The model under review builds one solid part; all positions refer to its coordinate system, in mm. Coordinates: 2 decimals unless noted, no trailing zeros. Order: outer loops, then holes, each group sorted by start corner. A loop starts at its lowest first (then second) coordinate and runs counter-clockwise, first axis right, second up. Notation, with made-up numbers: (42, -36.5) - (76, -36.5) arc R19 ccw to (76, -14.5) - close; hole circle Ø2 at (86, 60.5). An arc over 180 degrees is marked (long way). Answer in a Markdown table with one row per item.
```python
from build123d import *

# Parameters (mm, degrees)
F0_R        = 2.286
F1_DEPTH    = 8
F2_R        = 4
F3_R        = 4
F4_T1_DEPTH = 27.7658164516
F5_T1_DEPTH = 27.7658164516


# Not quite as in the source:
# - a fillet or chamfer that OpenCascade refuses, or shapes differently, is made with other operations: its cross-section is extruded or revolved along the edge and cut away or added


with BuildPart() as f1:
    # F0 (on Top) → F1 (new body)
    with BuildSketch(Plane.XY):
        Polygon((19.2099873261, 3.0477390712), (-18.8900126739, 3.0477390712), (-18.8900126739, -3.3271788533), (-17.4405010572, -3.3022609288), (19.2099873261, -3.3022609288), align=None)
        with Locations((-15.8400126739, -0.1272609288)):
            Circle(F0_R, mode=Mode.SUBTRACT)
        with Locations((-7.8400126739, -0.1272609288)):
            Circle(F0_R, mode=Mode.SUBTRACT)
        with Locations((0.1599873261, -0.1272609288)):
            Circle(F0_R, mode=Mode.SUBTRACT)
        with Locations((8.1599873261, -0.1272609288)):
            Circle(F0_R, mode=Mode.SUBTRACT)
        with Locations((16.1599873261, -0.1272609288)):
            Circle(F0_R, mode=Mode.SUBTRACT)
    extrude(amount=F1_DEPTH)

    # F2
    f2_edges = [f1.edges().sort_by_distance(p)[0] for p in [
        (-18.890013, -3.327179, 4),
    ]]
    fillet(f2_edges, radius=F2_R)

    # F3
    f3_edges = [f1.edges().sort_by_distance(p)[0] for p in [
        (19.209987, -3.302261, 4),
    ]]
    fillet(f3_edges, radius=F3_R)

    # F4: fillet of radius 4.5 on 1 edges, made by hand

    # F4_s2 → F4_t1 (cut)
    with BuildSketch(Plane.XY.offset(-9.8829082258)):
        with BuildLine():
            ThreePointArc((19.2099873261, 0.6977390712), (17.5562804933, 2.4158781586), (15.2568240358, 3.0477390712))
            Line((15.2568240358, 3.0477390712), (19.2099873261, 3.0477390712))
            Line((19.2099873261, 3.0477390712), (19.2099873261, 0.6977390712))
        make_face()
    extrude(amount=F4_T1_DEPTH, mode=Mode.SUBTRACT)

    # F5: fillet of radius 4.5 on 1 edges, made by hand

    # F5_s2 → F5_t1 (cut)
    with BuildSketch(Plane.XY.offset(-9.8829082258)):
        with BuildLine():
            ThreePointArc((-18.8900126739, 0.6977390712), (-17.2363058411, 2.4158781586), (-14.9368493836, 3.0477390712))
            Line((-14.9368493836, 3.0477390712), (-18.8900126739, 3.0477390712))
            Line((-18.8900126739, 3.0477390712), (-18.8900126739, 0.6977390712))
        make_face()
    extrude(amount=F5_T1_DEPTH, mode=Mode.SUBTRACT)


solid = f1.part
```
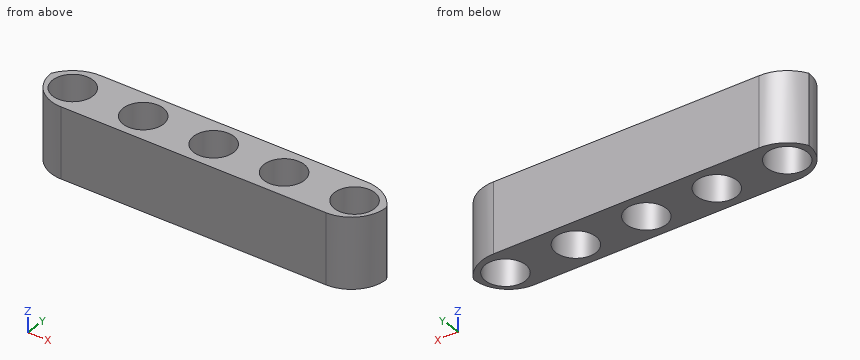
Item 1: We need section B-B, the plane x = -14. Write out the cut boundary in (y, z).
Check values:
| item | result |
|---|---|
| outline | (-3.3, 0) - (-1.48, 0) - (-1.48, 8) - (-3.3, 8) - close; (1.23, 0) - (3.05, 0) - (3.05, 8) - (1.23, 8) - close |
Item 2: We need section C-C, the plane z = 5.5. State how many separate pieces and enclosed holes the cut face has, then the cut area to 3 significant figures.
Check values:
| item | result |
|---|---|
| separate pieces | 1 |
| enclosed holes | 5 |
| area | 148 mm^2 |
Item 3: To check wall thickness, follow line 1 (X direction, y = -1.5, z = 4.75); line 2 (X direction, y = -1.75, z = 5.25); line 3 (Y direction, x = -8, z = 4.5). State the ranges of each line that lie inside material, in increasing order. Write a range as from..to.
Check values:
| item | result |
|---|---|
| line 1 | -18.23..-17.67, -14.01..-9.67, -6.01..-1.67, 1.99..6.33, 9.99..14.33, 17.99..18.55 |
| line 2 | -18.05..-17.45, -14.23..-9.45, -6.23..-1.45, 1.77..6.55, 9.77..14.55, 17.77..18.37 |
| line 3 | -3.3..-2.41, 2.15..3.05 |
Item 4: We need section A-A, the plane y = 1.25. Write out the cut boundary in (x, z).
Check values:
| item | result |
|---|---|
| outline | (-18.54, 0) - (-17.66, 0) - (-17.66, 8) - (-18.54, 8) - close; (-14.02, 0) - (-9.66, 0) - (-9.66, 8) - (-14.02, 8) - close; (-6.02, 0) - (-1.66, 0) - (-1.66, 8) - (-6.02, 8) - close; (1.98, 0) - (6.34, 0) - (6.34, 8) - (1.98, 8) - close; (9.98, 0) - (14.34, 0) - (14.34, 8) - (9.98, 8) - close; (17.98, 0) - (18.86, 0) - (18.86, 8) - (17.98, 8) - close |
Item 5: Clearance check with flat-ended pins moving along their axes: pin 1 Ø1 at (x, y) = (13.5, -0.5) entering from -Z; pin 2 Ø3 at (y, z) = (-1.5, 5) entering from -X. State where each tip first meets the part, or that it passes through.
Check values:
| item | result |
|---|---|
| pin 1 | z = 0 |
| pin 2 | x = -18.83 |
